Source: CAD feature listing. Evaluate the final solid. Frame: model axes, mm. Give positions to 0.01 mm unless a question says otherwise; leave off trailing zeros. Write each loop counter-clockwise with the first axis right and the second up, starting at its lowest first coordinate (ties: lowest second). Pieces come first, ordered by that corner, then holes. Notation, with made-up numbers: (-9, 37) -> (-3, 37) arc R26 cw to (-3, 61) -> close; hole circle Ø10 at (1, 63.25). An arc over 180 degrees is marked (long way). Use a Markdown table: item, result. Add a question column.
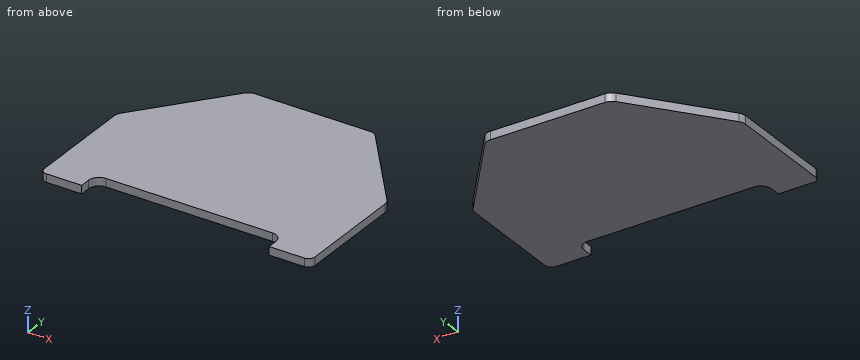
```python
from build123d import *

# Parameters (mm, degrees)
BOSS_EXTRUDE2_DEPTH = 3.95
FILLET1_R           = 5
FILLET2_R           = 3


with BuildPart() as part:
    # Sketch1 → Boss-Extrude2 (new body)
    with BuildSketch(Plane.XY):
        Polygon((0, 56), (35, 100), (95, 100), (130, 56), (130, 0), (110, 0), (110, 10), (20, 10), (20, 0), (0, 0), align=None)
    extrude(amount=BOSS_EXTRUDE2_DEPTH)

    # Fillet1
    fillet1_edges = [part.edges().sort_by_distance(p)[0] for p in [
        (110, 10, 1.975),
        (20, 10, 1.975),
        (0, 56, 1.975),
        (35, 100, 1.975),
        (95, 100, 1.975),
        (130, 56, 1.975),
    ]]
    fillet(fillet1_edges, radius=FILLET1_R)

    # Fillet2
    fillet2_edges = [part.edges().sort_by_distance(p)[0] for p in [
        (0, 0, 1.975),
        (130, 0, 1.975),
    ]]
    fillet(fillet2_edges, radius=FILLET2_R)


solid = part.part
```
(1) Material intervals for L1, parallel to Y at x = 73, z = 0.5; L2, parallel to Y at x = 15, z = 3.35; L3, parallel to X at y = 60.5, z = 0.25, sorted ascending.
(2) First-contact query: pin 1 Ø1.2 at (x, z) = (63.5, 2.5) entering from -Y; pin 2 Ø1.2 at (y, z) = (2, 1) entering from -X; pin 3 Ø1.5 at (x, z) = (103.5, 0.5) entering from +Y. Flat tips, straight axial feed; report the tip coordinate or a pass-through.
(3) Cut plane C-C on y = 81. Return the cut outline in (x, z), then the cut area to 3 significant figures.
(4) Cut plane A-A on z = 0.7. Return the cut outline in (x, y), then the cut area to 3 significant figures.
(5) Cut plane B-B on x = 65. Return the cut outline in (y, z).
Output:
| question | item | result |
|---|---|---|
| 1 | L1 | 10 to 100 |
| 1 | L2 | 0 to 74.86 |
| 1 | L3 | 3.58 to 126.42 |
| 2 | pin 1 | y = 10 |
| 2 | pin 2 | x = 0.03 |
| 2 | pin 3 | y = 90.26 |
| 3 | outline | (19.89, 0) -> (110.11, 0) -> (110.11, 3.95) -> (19.89, 3.95) -> close |
| 3 | area | 356 mm^2 |
| 4 | outline | (0, 3) arc R3 ccw to (3, 0) -> (20, 0) -> (20, 5) arc R5 cw to (25, 10) -> (105, 10) arc R5 cw to (110, 5) -> (110, 0) -> (127, 0) arc R3 ccw to (130, 3) -> (130, 54.25) arc R5 ccw to (128.91, 57.37) -> (96.5, 98.11) arc R5 ccw to (92.59, 100) -> (37.41, 100) arc R5 ccw to (33.5, 98.11) -> (1.09, 57.37) arc R5 ccw to (0, 54.25) -> close |
| 4 | area | 10,600 mm^2 |
| 5 | outline | (10, 0) -> (100, 0) -> (100, 3.95) -> (10, 3.95) -> close |
